```python
from build123d import *

# Parameters (mm, degrees)
EXTRUDE_1_DEPTH          = 30
CUT_EXTRUDE_1_DEPTH      = 98.124713642
CUT_EXTRUDE_1_DEPTH_BACK = 98.124713642
SKETCH_2_R               = 1.5
CUT_EXTRUDE_6_DEPTH      = 10
EXTRUDE_3_DEPTH          = 12.5
SKETCH_12_W              = 5
SKETCH_12_H              = 30
EXTRUDE_4_DEPTH          = 2
SKETCH_17_W              = 25
SKETCH_17_H              = 25
EXTRUDE_7_DEPTH          = 40
CUT_EXTRUDE_9_DEPTH      = 50
SKETCH_21_R              = 1.5
CUT_EXTRUDE_12_DEPTH     = 7
CUT_EXTRUDE_13_DEPTH     = 500
SKETCH_23_W              = 17
SKETCH_23_H              = 21
CUT_EXTRUDE_14_DEPTH     = 4


with BuildPart() as part:
    # 草图1 → 凸台-拉伸1 (new body)
    with BuildSketch(Plane(origin=(0, 0, 0), x_dir=(1, 0, 0), z_dir=(0, 1, 0))):
        with BuildLine():
            Line((0, 0), (-70, 0))
            ThreePointArc((-70, 0), (-41.606545869, -31.737243891), (-10, -60.276114672))
            Line((-10, -60.276114672), (-10, -15))
            Line((-10, -15), (0, -15))
            Line((0, -15), (0, -10))
            Line((0, -10), (-10, -10))
            Line((-10, -10), (-10, -5))
            Line((-10, -5), (0, -5))
            Line((0, -5), (0, 0))
        make_face()
    extrude(amount=EXTRUDE_1_DEPTH)

    # 草图2 → 切除-拉伸1 (cut, two sides: drawn at the far end of the back side and taken through both)
    with BuildSketch(Plane(origin=(0, 0, 0), x_dir=(-1, 0, 0), z_dir=(0, 0, -1)).offset(-CUT_EXTRUDE_1_DEPTH_BACK)):
        with Locations((4, 25)):
            Circle(SKETCH_2_R)
        with Locations((4, 5)):
            Circle(SKETCH_2_R)
    extrude(amount=CUT_EXTRUDE_1_DEPTH + CUT_EXTRUDE_1_DEPTH_BACK, mode=Mode.SUBTRACT)

    # 草图9 → 切除-拉伸6 (cut, symmetric)
    with BuildSketch(Plane(origin=(0, 15, 0), x_dir=(1, 0, 0), z_dir=(0, 1, 0))):
        with BuildLine():
            Line((-65.918016471, -5), (-59.391772218, -5))
            Line((-59.391772218, -5), (-15, -5))
            Line((-15, -5), (-15, -15))
            Line((-15, -15), (-15, -49.60330608))
            Line((-15, -49.60330608), (-15, -56.155472209))
            ThreePointArc((-15, -56.155472209), (-41.615194331, -31.728555364), (-65.918016471, -5))
        make_face()
    extrude(amount=CUT_EXTRUDE_6_DEPTH, both=True, mode=Mode.SUBTRACT)

    # 草图11 → 凸台-拉伸3 (add, symmetric)
    with BuildSketch(Plane(origin=(0, 15, 0), x_dir=(1, 0, 0), z_dir=(0, 1, 0))):
        Polygon((-15, -5), (-23, -5), (-15, -10), align=None)
    extrude(amount=EXTRUDE_3_DEPTH, both=True)

    # 草图12 → 凸台-拉伸4 (add)
    with BuildSketch(Plane(origin=(0, 0, 0), x_dir=(0, 0, -1), z_dir=(1, 0, 0))):
        with Locations((-12.5, 15)):
            Rectangle(SKETCH_12_W, SKETCH_12_H)
        with Locations((-2.5, 15)):
            Rectangle(SKETCH_12_W, SKETCH_12_H)
    extrude(amount=EXTRUDE_4_DEPTH)

    # 草图17 → 凸台-拉伸7 (add)
    with BuildSketch(Plane.XZ):
        with Locations((-32.5, 12.5)):
            Rectangle(SKETCH_17_W, SKETCH_17_H)
    extrude(amount=EXTRUDE_7_DEPTH)

    # 草图18 → 切除-拉伸9 (cut)
    with BuildSketch(Plane.ZY.offset(45)):
        Polygon((0, 0), (25, -40), (0, -40), align=None)
    extrude(amount=-CUT_EXTRUDE_9_DEPTH, mode=Mode.SUBTRACT)

    # 草图21 → 切除-拉伸12 (cut)
    with BuildSketch(Plane(origin=(0, 0, 0), x_dir=(-1, 0, 0), z_dir=(0, -0.52999894000318, -0.8479983040050879))):
        with Locations(Location((32.5, -22.16990566, 0), (0, 0, 90))):
            Circle(SKETCH_21_R)
        with Locations(Location((32.5, -12.16990566, 0), (0, 0, 90))):
            Circle(SKETCH_21_R)
        with Locations(Location((32.5, -32.16990566, 0), (0, 0, 90))):
            Circle(SKETCH_21_R)
    extrude(amount=-CUT_EXTRUDE_12_DEPTH, mode=Mode.SUBTRACT)

    # 草图22 → 切除-拉伸13 (cut)
    with BuildSketch(Plane.ZY.offset(45)):
        Polygon((7.216990566, -4), (21, -4), (21, -26.052815094), align=None)
    extrude(amount=-CUT_EXTRUDE_13_DEPTH, mode=Mode.SUBTRACT)

    # 草图23 → 切除-拉伸14 (cut)
    with BuildSketch(Plane.XY.offset(25)):
        with Locations((-32.5, -14.5)):
            Rectangle(SKETCH_23_W, SKETCH_23_H)
    extrude(amount=-CUT_EXTRUDE_14_DEPTH, mode=Mode.SUBTRACT)


solid = part.part
```
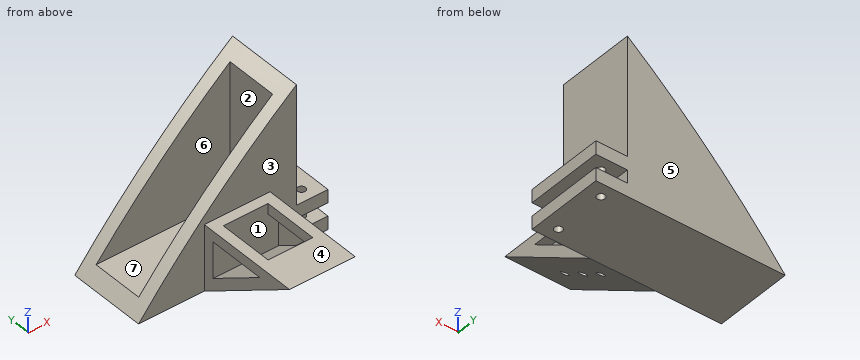
Model file for the job. Use its own axes, mm. Face numbers are marked on the shaded views. A direction names the side the tool comes from. Coordinates: 2 decimals unless noted, no trailing zeros. Write each loop counter-clockwise with the first axis right and the second up, starting at its lowest first coordinate (ties: lowest second). Pieces come first, ordered by that corner, then holes. Notation, with made-up numbers: (-13.5, 10) - (18.5, 10) arc R23 cw to (18.5, 23) - close; hole circle Ø7 at (-37, 60). An arc over 180 degrees is marked (long way). One line per item, written item: value. Start each with the question number.
1. Slice it at C-C (z = 35). Write the cut outline in (x, y), plus the area to 3 significant figures.
2. Mould opens along Y. For the marked faces 4, 5, 6 and 7 say: released by +Y, released by -Y, zero draft, split by the parting line, or undercut.
3. Slice it at B-B (y = -5). Write the cut outline in (x, z) (3 decimals), plus the area to 3 significant figures.
4. Slice it at D-D (x = -21). Write the cut outline in (y, z), plus the area to 3 significant figures.
5. Flat gauge pins, fed straight in: pin 1 (1.5 mm diameter, centred on y = 9, z = 7.5, fed in from +X); pin 2 (2 mm diameter, centred on y = -20, z = 15, fed in from +X); pin 3 (12.5 mm diameter, centred on x = -26.5, y = -18, fed in from -Z). Where does each tip first touch, or does it go through?
6. Probe line 1 (Y direction, x = -4, z = 2); line 2 (Y direction, x = -23.5, z = 34.5); line 3 (X direction, y = -9, z = 22.5). List the from-to ranges inside material, lowest first. Write a range as from..to.
7. Slice it at A-A (x = -4). Write the cut outline in (y, z).
8. Tool access for the marked faces 1, 2 and 3: list every direction of +Z, -Z, +X, -X, +Y, -Y with a clear straight run to the whole face (end or side of a thin tool).
Answers below:
1. outline: (-38.32, 0) - (-10, 0) - (-10, 30) - (-38.32, 30) - (-38.32, 25) - (-15, 25) - (-15, 5) - (-38.32, 5) - close
1. area: 383 mm^2
2. face 4: zero draft
2. face 5: released by +Y
2. face 6: undercut
2. face 7: undercut
3. outline: (-45, 3.125) - (-20, 3.125) - (-20, 7.842) - (-45, 7.842) - close; (-45, 21) - (-41, 21) - (-41, 25) - (-45, 25) - close; (-24, 21) - (-20, 21) - (-20, 25) - (-24, 25) - close
3. area: 150 mm^2
4. outline: (-40, 25) - (0, 0) - (30, 0) - (30, 51.03) - (25, 51.03) - (25, 6.25) - (5, 6.25) - (5, 51.03) - (0, 51.03) - (0, 25) - close; hole (-26.05, 21) - (-4, 7.22) - (-4, 21) - close
4. area: 983 mm^2
5. pin 1: stops at x = -10
5. pin 2: stops at x = -20
5. pin 3: stops at z = 7.34
6. line 1: y = 0..3.5, 6.5..23.5, 26.5..30
6. line 2: y = 0..5, 25..30
6. line 3: x = -45..-41, -24..-20
7. outline: (0, 0) - (3.5, 0) - (3.5, 5) - (0, 5) - close; (0, 10) - (3.5, 10) - (3.5, 15) - (0, 15) - close; (6.5, 0) - (23.5, 0) - (23.5, 5) - (6.5, 5) - close; (6.5, 10) - (23.5, 10) - (23.5, 15) - (6.5, 15) - close; (26.5, 0) - (30, 0) - (30, 5) - (26.5, 5) - close; (26.5, 10) - (30, 10) - (30, 15) - (26.5, 15) - close
8. face 1: none
8. face 2: +Z, -X
8. face 3: +Z, -Y
